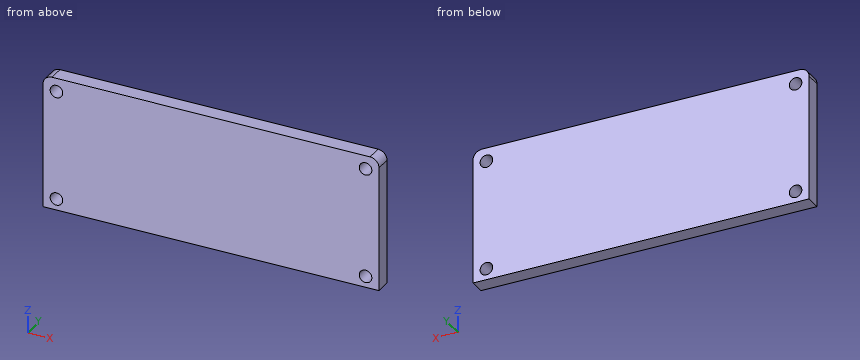
from build123d import *

# Parameters (mm, degrees)
SKETCH1_W                   = 190.5
SKETCH1_H                   = 76.2
BOSS_EXTRUDE1_DEPTH         = 8.89
F_1_4_CLEARANCE_HOLE1_D     = 7.14248
F_1_4_CLEARANCE_HOLE1_DEPTH = 8.89
FILLET1_R                   = 5.08


with BuildPart() as part:
    # Sketch1 → Boss-Extrude1 (new body)
    with BuildSketch(Plane(origin=(0, 0, 0), x_dir=(1, 0, 0), z_dir=(0, 1, 0))):
        Rectangle(SKETCH1_W, SKETCH1_H)
    extrude(amount=BOSS_EXTRUDE1_DEPTH)

    # 1/4 Clearance Hole1
    with Locations(Plane(origin=(0, 8.89, 0), x_dir=(-1, 0, 0), z_dir=(0, 1, 0))):
        with Locations((87.63, -31.75), (-87.63, -31.75), (-87.63, 30.48), (87.63, 30.48)):
            Hole(F_1_4_CLEARANCE_HOLE1_D / 2, depth=F_1_4_CLEARANCE_HOLE1_DEPTH)

    # Fillet1
    fillet1_edges = [part.edges().sort_by_distance(p)[0] for p in [
        (95.25, 4.445, 38.1),
        (-95.25, 4.445, 38.1),
    ]]
    fillet(fillet1_edges, radius=FILLET1_R)


solid = part.part
Build history of the part. All positions in model axes, mm. Round coordinates to 2 decimals unless told otherwise and drop trailing zeros. Write each loop counter-clockwise with the first axis right and the second up, starting at its lowest first coordinate (ties: lowest second). Pieces come first, ordered by that corner, then holes. Notation, with made-up numbers: (69.25, 7) -> (107.25, 7) arc R5 ccw to (107.25, 16) -> close; hole circle Ø3 at (26, -18). An arc over 180 degrees is marked (long way). Write item = value, one per line.
(1) Band-saw the part on B-B (x = -87.63). Give the cut face in (y, z), then the cut area to 3 significant figures.
Answer:
outline = (0, -38.1) -> (8.89, -38.1) -> (8.89, -35.32) -> (0, -35.32) -> close; (0, -28.18) -> (8.89, -28.18) -> (8.89, 26.91) -> (0, 26.91) -> close; (0, 34.05) -> (8.89, 34.05) -> (8.89, 38.1) -> (0, 38.1) -> close
area = 550 mm2
(2) Probe L1, parallel to Z at x = 87.63, y = 2.25; L2, parallel to X at y = 1.5, z = -31. List the from-to ranges inside material, lowest first.
Answer:
L1 = -38.1 to -35.32, -28.18 to 26.91, 34.05 to 38.1
L2 = -95.25 to -91.12, -84.14 to 84.14, 91.12 to 95.25
(3) Band-saw the part on A-A (z = 30.48). Give the cut face in (x, y), then the cut area to 3 significant figures.
Answer:
outline = (-95.25, 0) -> (-91.2, 0) -> (-91.2, 8.89) -> (-95.25, 8.89) -> close; (-84.06, 0) -> (84.06, 0) -> (84.06, 8.89) -> (-84.06, 8.89) -> close; (91.2, 0) -> (95.25, 0) -> (95.25, 8.89) -> (91.2, 8.89) -> close
area = 1,570 mm2
